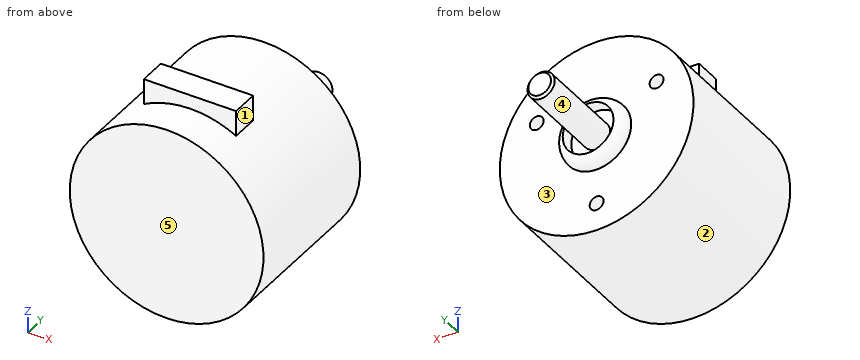
from build123d import *

# Parameters (mm, degrees)
SKETCH1_R           = 21
SKETCH1_R_2         = 1.5
SKETCH1_R_3         = 7.5
SKETCH1_R_4         = 5.5
SKETCH1_R_5         = 2.945
BOSS_EXTRUDE1_DEPTH = 17
CUT_EXTRUDE1_START  = 17
SKETCH1_3_R         = 1.5
CUT_EXTRUDE1_DEPTH  = 10
BOSS_EXTRUDE2_START = 17
SKETCH1_4_R         = 7.5
SKETCH1_4_R_2       = 5.5
BOSS_EXTRUDE2_DEPTH = 3
FILLET1_R           = 3
BOSS_EXTRUDE3_START = 17
SKETCH1_5_R         = 2.945
BOSS_EXTRUDE3_DEPTH = 20
BOSS_EXTRUDE4_START = -2.8
BOSS_EXTRUDE4_DEPTH = 6
CHAMFER1_SIZE       = 0.5


with BuildPart() as part:
    # Sketch1 → Boss-Extrude1 (new, symmetric)
    # profile 1 of 7: a face of its own
    with BuildSketch(Plane(origin=(0, 0, 0), x_dir=(1, 0, 0), z_dir=(0, 1, 0))):
        with Locations(Location((0, 0, 0), (0, 0, 270))):
            Circle(SKETCH1_R)
        with Locations((12.990381057, -7.5)):
            Circle(SKETCH1_R_2, mode=Mode.SUBTRACT)
        with Locations((-12.990381057, -7.5)):
            Circle(SKETCH1_R_2, mode=Mode.SUBTRACT)
        with Locations((0, 15)):
            Circle(SKETCH1_R_2, mode=Mode.SUBTRACT)
        Circle(SKETCH1_R_3, mode=Mode.SUBTRACT)
    # profile 2 of 7: a face of its own
    with BuildSketch(Plane(origin=(0, 0, 0), x_dir=(1, 0, 0), z_dir=(0, 1, 0))):
        Circle(SKETCH1_R_3)
        Circle(SKETCH1_R_4, mode=Mode.SUBTRACT)
    # profile 3 of 7: a face of its own
    with BuildSketch(Plane(origin=(0, 0, 0), x_dir=(1, 0, 0), z_dir=(0, 1, 0))):
        Circle(SKETCH1_R_4)
        Circle(SKETCH1_R_5, mode=Mode.SUBTRACT)
    # profile 4 of 7: a face of its own
    with BuildSketch(Plane(origin=(0, 0, 0), x_dir=(1, 0, 0), z_dir=(0, 1, 0))):
        Circle(SKETCH1_R_5)
    # profile 5 of 7: a face of its own
    with BuildSketch(Plane(origin=(0, 0, 0), x_dir=(1, 0, 0), z_dir=(0, 1, 0))):
        with Locations((-12.990381057, -7.5)):
            Circle(SKETCH1_R_2)
    # profile 6 of 7: a face of its own
    with BuildSketch(Plane(origin=(0, 0, 0), x_dir=(1, 0, 0), z_dir=(0, 1, 0))):
        with Locations((12.990381057, -7.5)):
            Circle(SKETCH1_R_2)
    # profile 7 of 7: a face of its own
    with BuildSketch(Plane(origin=(0, 0, 0), x_dir=(1, 0, 0), z_dir=(0, 1, 0))):
        with Locations((0, 15)):
            Circle(SKETCH1_R_2)
    extrude(amount=BOSS_EXTRUDE1_DEPTH, both=True)

    # Sketch1<3> → Cut-Extrude1 (cut)
    with BuildSketch(Plane(origin=(0, 0, 0), x_dir=(1, 0, 0), z_dir=(0, 1, 0)).offset(CUT_EXTRUDE1_START)):
        with Locations(Location((-12.990381057, -7.5, 0), (0, 0, 270))):
            Circle(SKETCH1_3_R)
        with Locations(Location((12.990381057, -7.5, 0), (0, 0, 270))):
            Circle(SKETCH1_3_R)
        with Locations(Location((0, 15, 0), (0, 0, 270))):
            Circle(SKETCH1_3_R)
    extrude(amount=-CUT_EXTRUDE1_DEPTH, mode=Mode.SUBTRACT)

    # Sketch1<4> → Boss-Extrude2 (add)
    with BuildSketch(Plane(origin=(0, 0, 0), x_dir=(1, 0, 0), z_dir=(0, 1, 0)).offset(BOSS_EXTRUDE2_START)):
        with Locations(Location((0, 0, 0), (0, 0, 270))):
            Circle(SKETCH1_4_R)
        with Locations(Location((0, 0, 0), (0, 0, 270))):
            Circle(SKETCH1_4_R_2, mode=Mode.SUBTRACT)
    extrude(amount=BOSS_EXTRUDE2_DEPTH)

    # Fillet1
    # the kernel refuses this fillet: 3 mm, written as the material it takes off along each edge
    with BuildSketch(Plane(origin=(0, 20, 0), x_dir=(0, 0, 1), z_dir=(-1, 0, 0))) as fillet1_piece_1:
        with BuildLine():
            CenterArc((4.5, -2.828427125), FILLET1_R, 0, 70.528779366)
            Line((5.5, 0), (5.52, 0.056568542))
            ThreePointArc((5.52, 0.056568542), (6.5, 0.06), (7.5, 0.06))
            Line((7.5, 0.06), (7.56, 0))
            Line((7.56, 0), (7.56, -2.828427125))
            Line((7.56, -2.828427125), (7.5, -2.828427125))
        make_face()
    revolve(axis=Axis((0, 20, 0), (0, 1, 0)), mode=Mode.SUBTRACT)

    # Sketch1<5> → Boss-Extrude3 (add)
    with BuildSketch(Plane(origin=(0, 0, 0), x_dir=(1, 0, 0), z_dir=(0, 1, 0)).offset(BOSS_EXTRUDE3_START)):
        with Locations(Location((0, 0, 0), (0, 0, 270))):
            Circle(SKETCH1_5_R)
    extrude(amount=BOSS_EXTRUDE3_DEPTH)

    # Sketch1<8> → Boss-Extrude4 (add)
    with BuildSketch(Plane(origin=(0, 0, 0), x_dir=(1, 0, 0), z_dir=(0, 1, 0)).offset(BOSS_EXTRUDE4_START)):
        with BuildLine():
            ThreePointArc((10, -18.466185313), (0, -21), (-10, -18.466185313))
            Line((-10, -18.466185313), (-10, -24))
            Line((-10, -24), (10, -24))
            Line((10, -24), (10, -18.466185313))
        make_face()
    extrude(amount=-BOSS_EXTRUDE4_DEPTH)

    # Chamfer1
    chamfer1_edges = [part.edges().sort_by_distance(p)[0] for p in [
        (0, 37, -2.945),
    ]]
    chamfer(chamfer1_edges, length=CHAMFER1_SIZE)


solid = part.part
The model under review builds one solid part; all positions refer to its coordinate system, in mm. Face numbers are marked on the shaded views. A direction names the side the tool comes from. Give positions to 0.01 mm unless a question says otherwise; leave off trailing zeros. Order: outer loops, then holes, each group sorted by start corner. A loop starts at its lowest first (then second) coordinate and runs counter-clockwise, first axis right, second up. Notation, with made-up numbers: M 48,10 L 74,10 A9 ccw 74,17 Z; hole C 65,-39 d9. An arc over 180 degrees is marked long. Use one line per item in the form item = value. Start each with the question number.
Item 1: The part is to be moulded in two halves that separate along X. For the marked faces 1, 2 and 3, say which applies: pulls with the +X half, pulls with the -X half, needs draft (parallel to the pull), parting line crosses it, or undercut.
Item 2: We need section B-B on x = 0. Give the boundary of the cut face in (y, z) (3 decimals).
Item 3: For the marked faces 4 and 5, list the 3-axis set-ups (+Z, -Z, +X, -X, +Y, -Y) from which the entire face can be reached by the end or side of a thin tool; tool diameter is ignored.
Item 4: Insertion check: pin 1 Ø4.5 at (y, z) = (-4.5, 22) entering from -X; pin 2 Ø3.5 at (x, z) = (-13.5, 7) entering from +Y; pin 3 Ø12 at (y, z) = (-7.5, 11.5) entering from +X. Each pin has a flat end and moves straight along its axis. Give the tip position at first contact, or say it passes through.
Item 5: To check wall thickness, follow line 1 along Y through (x, z) = (0, 14.5); line 2 along X through (y, z) = (12.25, 7.5); line 3 along X through (y, z) = (18.5, 0) (3 decimals). State the ranges of each line that lie inside material, in increasing order. Write a range as from..to.
Item 6: We need section A-A on z = 0. Give the boundary of the cut face in (x, y) (3 decimals).
Item 7: We need section D-D on y = 13. Give the boundary of the cut face in (x, z).
Item 8: We need section C-C on y = 33.5. Give the boundary of the cut face in (x, z) (3 decimals), plus the area to 3 significant figures.
Completed:
q1.face_1 = pulls with the +X half
q1.face_2 = parting line crosses it
q1.face_3 = needs draft
q2.outline = M -17,-21 L 17,-21 L 17,-16.5 L 7,-16.5 L 7,-13.5 L 17,-13.5 L 17,-7.5 L 17.172,-7.5 A3 ccw 20,-5.5 L 17,-5.5 L 17,-2.945 L 36.5,-2.945 L 37,-2.445 L 37,2.445 L 36.5,2.945 L 17,2.945 L 17,5.5 L 20,5.5 A3 ccw 17.172,7.5 L 17,7.5 L 17,21 L -2.8,21 L -2.8,24 L -8.8,24 L -8.8,21 L -17,21 Z
q3.face_4 = +Y
q3.face_5 = +Z, -Z, +X, -X, -Y
q4.pin_1 = -10
q4.pin_2 = 17
q4.pin_3 = 20.27
q5.line_1 = -17..17
q5.line_2 = -19.62..-14.49, -11.49..11.49, 14.49..19.62
q5.line_3 = -7.19..-5.5, -2.945..2.945, 5.5..7.19
q6.outline = M -21,-17 L 21,-17 L 21,17 L 7.5,17 L 7.5,17.172 A3 ccw 5.5,20 L 5.5,17 L 2.945,17 L 2.945,36.5 L 2.445,37 L -2.445,37 L -2.945,36.5 L -2.945,17 L -5.5,17 L -5.5,20 A3 ccw -7.5,17.172 L -7.5,17 L -21,17 Z
q7.outline = C 0,0 d42; hole C -12.99,7.5 d3; hole C 0,-15 d3; hole C 12.99,7.5 d3
q8.outline = C 0,0 d5.89
q8.area = 27.2 mm²
